Geometry check sheet. Reference: drawing and pictorial views, mm from the part's lowest x, y, z. A direction names the side the tool comes from. Coordinates: 2 decimals unless noted, no trailing zeros. Write each loop counter-clockwise with the first axis right and the second up, starting at its lowest first coordinate (ties: lowest second). Pieces come first, ordered by that corner, then holes. Notation, with made-up numbers: M 19.5,89.25 L 69.5,89.25 A12 ccw 69.5,108.25 Z; hole C 0.25,38.5 d2. An arc over 180 degrees is marked long. One line per item, written item: value.
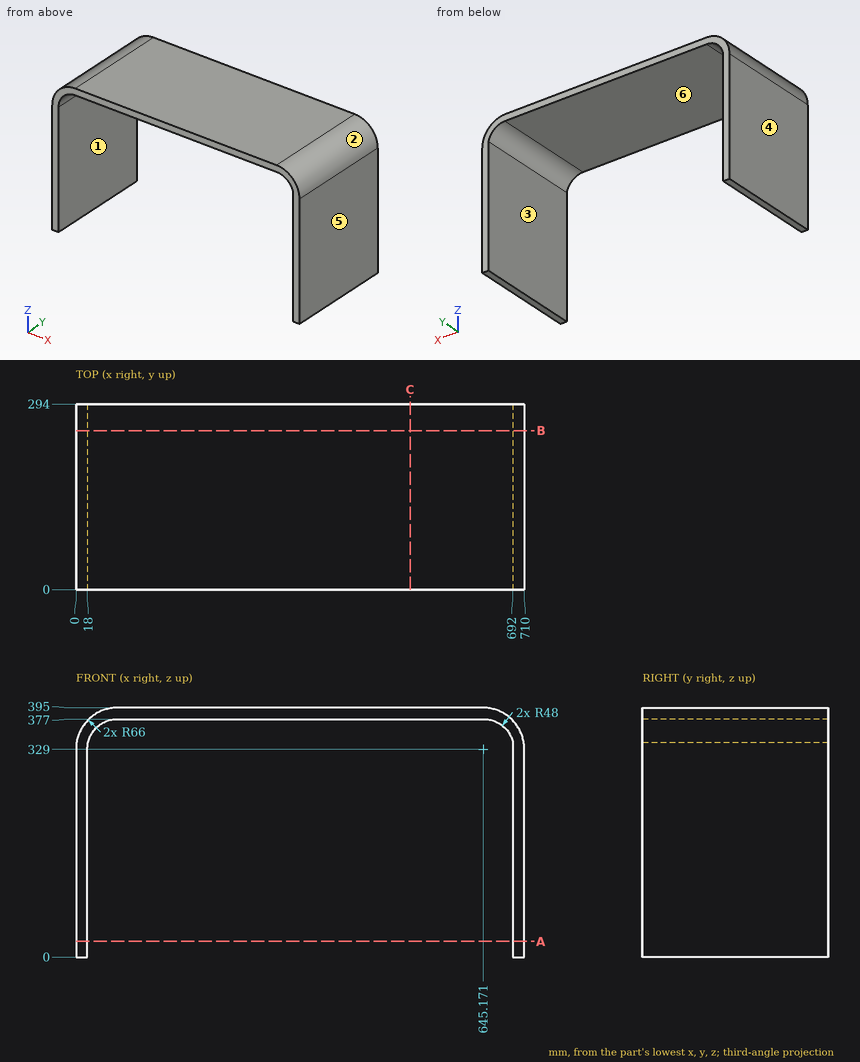
Item 1: Draft check along X on the marked faces 1, 2, 3 and 4. Enter one of: released by +X, released by -X, zero draft, split by the parting line, or undercut.
The answers:
face 1: undercut
face 2: released by +X
face 3: undercut
face 4: released by -X
Item 2: Cross-section at A-A, the plane z = 25. Enter the section's corners in (x, y), and give its area (3 significant figures).
The answers:
outline: M 0,0 L 18,0 L 18,294 L 0,294 Z; M 692,0 L 710,0 L 710,294 L 692,294 Z
area: 10,600 mm²
Item 3: Go/stop test with a flat-tipped pin: P1, Ø1, axis at x = 100.5, y = 236, coming from the -Z side. Record where the tip stops, or that it passes through.
The answers:
P1: stops at z = 377
Item 4: Cross-section at B-B, the plane y = 252. Enter the section's corners in (x, z).
The answers:
outline: M 0,0 L 18,0 L 18,329 A48 cw 66,377 L 645.17,377 A48 cw 692,339.54 L 692,0 L 710,0 L 710,329 A66 ccw 644,395 L 66,395 A66 ccw 0,329 Z
Item 5: Cross-section at C-C, the plane x = 529. Enter the section's corners in (y, z), and give its area (3 significant figures).
The answers:
outline: M 0,377 L 294,377 L 294,395 L 0,395 Z
area: 5,290 mm²
Item 6: Scan lines: line 1 (X direction, y = 80.5, z = 83); line 2 (Z direction, x = 582, y = 198.5); line 3 (Z direction, x = 675, y = 100) (1 decimal). Record each from-to range of solid material in increasing order.
The answers:
line 1: x = 0 to 18, 692 to 710
line 2: z = 377 to 395
line 3: z = 366.6 to 387.3
Item 7: Access from +Z, -Z, +X, -X, +Y, -Y to the whole of each face (thin tool, end or side, straight path). Record for the marked faces 5 and 6.
The answers:
face 5: +Z, -Z, +X, +Y, -Y
face 6: -Z, +Y, -Y
